Could you check a few things on this model? Use its own coordinates, in mm. Coordinates: 2 decimals unless noted, no trailing zeros. Order: outer loops, then holes, each group sorted by start corner. A loop starts at its lowest first (then second) coordinate and runs counter-clockwise, first axis right, second up. Notation, with made-up numbers: (26, 74) -> (54, 74) arc R23 cw to (54, 109) -> close; hole circle Ø8 at (3, 54). An arc over 180 degrees is marked (long way). Use a Markdown table: item, result. Add a question column.
1) If I drill on L1, parallel to Y at x = 5.08, z = 0.8; L2, parallel to Y at x = 4.5, z = 0.5; L3, parallel to Y at x = 21.08, z = 2.3, over which ranges is the centre line in solid material (lowest first)? Write a range as [from, to].
2) Will these pins go through, and if not, where does the flat tip stop? pin 1 Ø1 at (y, z) = (-2, 1.5) entering from -X; pin 2 Ø1 at (x, z) = (86, 1) entering from -Y.
3) If we section it at A-A (z = 2.4): Give the number of separate pieces and of enclosed holes in the cut face, plus the area to 3 significant figures.
4) If we section it at B-B (x = 31.5): Write out the boundary of the cut face in (y, z) (3 decimals), plus the area to 3 significant figures.
```python
from build123d import *

# Parameters (mm, degrees)
SKETCH1_R           = 2.8575
SKETCH1_R_2         = 0.75
BOSS_EXTRUDE1_DEPTH = 3.175
FILLET1_R           = 6.35


with BuildPart() as part:
    # Sketch1 → Boss-Extrude1 (new body)
    with BuildSketch(Plane.XY):
        Polygon((95.25, 0), (95.25, -3.175), (88.9, -3.175), (88.9, 0), (82.55, 0), (82.55, -3.175), (76.2, -3.175), (76.2, 0), (69.85, 0), (69.85, -3.175), (63.5, -3.175), (63.5, 0), (57.15, 0), (57.15, -3.175), (50.8, -3.175), (50.8, 0), (44.45, 0), (0, 0), (0, 25.4), (101.6, 25.4), (101.6, 0), align=None)
        with Locations((5.08, 5.08)):
            Circle(SKETCH1_R, mode=Mode.SUBTRACT)
        with Locations((5.08, 21.08)):
            Circle(SKETCH1_R_2, mode=Mode.SUBTRACT)
        with Locations((21.08, 5.08)):
            Circle(SKETCH1_R_2, mode=Mode.SUBTRACT)
    extrude(amount=BOSS_EXTRUDE1_DEPTH)

    # Fillet1
    fillet1_edges = [part.edges().sort_by_distance(p)[0] for p in [
        (101.6, 25.4, 1.5875),
    ]]
    fillet(fillet1_edges, radius=FILLET1_R)


solid = part.part
```
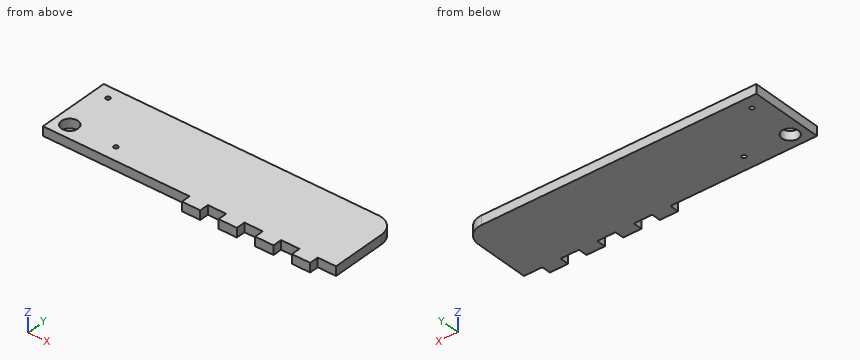
Answer sheet:
| question | item | result |
|---|---|---|
| 1 | L1 | [0, 2.22], [7.94, 20.33], [21.83, 25.4] |
| 1 | L2 | [0, 2.28], [7.88, 20.6], [21.56, 25.4] |
| 1 | L3 | [0, 4.33], [5.83, 25.4] |
| 2 | pin 1 | x = 50.8 |
| 2 | pin 2 | y = 0 |
| 3 | separate pieces | 1 |
| 3 | enclosed holes | 3 |
| 3 | area | 2,620 mm2 |
| 4 | outline | (0, 0) -> (25.4, 0) -> (25.4, 3.175) -> (0, 3.175) -> close |
| 4 | area | 80.6 mm2 |
